Design review of the part built by this model. Coordinates are the model's own, in mm. A direction names the side the tool comes from. Round coordinates to 2 decimals unless told otherwise and drop trailing zeros. Order: outer loops, then holes, each group sorted by start corner. A loop starts at its lowest first (then second) coordinate and runs counter-clockwise, first axis right, second up. Notation, with made-up numbers: M -9.75,29.5 L 33.25,29.5 A16 cw 33.25,46.5 Z; hole C 57,-23 d9. An arc over 180 degrees is marked long. Use a Markdown table: item, result. Add a question column.
(1) For pin 1 (1.3 mm diameter, centred on x = 19, z = 15, fed in from -Y); pin 2 (5 mm diameter, centred on y = -55, z = 13.5, fed in from -X); pin 3 (7 mm diameter, centred on y = -20, z = 6, fed in from -X), all flat-tipped, find the tip position at first contact; note any pin that passes through.
(2) Take a section at D-D (z = 1.5). Write out the cut boundary in (x, y).
(3) Take a section at A-A (z = 11.5). Write out the cut boundary in (x, y), then the cut area to 3 significant figures.
(4) To check wall thickness, follow probe 1 along X at (y, z) = (-6, 17.5); probe 2 along Y at (x, z) = (8, 9.25); probe 3 along Y at (x, z) = (19, 12.75). State the ranges of each line that lie inside material, in increasing order. Write a range as from..to.
(5) Take a section at B-B (x = -12). Write out the cut boundary in (y, z).
(6) Machinability: for faces 1 (the face through (-8.47, -48.65, 4.29)), 2 (the face through (10.631, -13, 11)), 3 (the face through (-33, 11.072, 11)), 4 (the face through (-35.89, 22.67, 11.34)), 5 (the face through (-7, 8, 23)), which of the approach directions +Z, -Z, +X, -X, +Y, -Y give a long, thin tool a straight path to every point of the face, cutting with its end or side? Answer none if there is none.
(7) Take a section at C-C (y = 9.5). Write out the cut boundary in (x, z).
```python
from build123d import *

# Parameters (mm, degrees)
F0_W     = 35
F0_H     = 40
F1_DEPTH = 23
F2_R     = 3
F3_R     = 4
F4_R     = 7
F5_R     = 7.384577
F6_DEPTH = 40


with BuildPart() as f1:
    # F0 (on Top) → F1 (new body)
    with BuildSketch(Plane.XY):
        with Locations((-6.869268, -8.927752)):
            Rectangle(F0_W, F0_H)
        Polygon((19.630732, 31.072248), (-33.369268, 31.072248), (-39.369268, 11.072248), (-24.369268, 11.072248), (10.630732, 11.072248), (25.630732, 11.072248), align=None)
    extrude(amount=F1_DEPTH)

    # F2
    f2_edges = [f1.edges().sort_by_distance(p)[0] for p in [
        (-33.369268, 31.072248, 11.5),
        (19.630732, 31.072248, 11.5),
    ]]
    fillet(f2_edges, radius=F2_R)

    # F3
    f3_edges = [f1.edges().sort_by_distance(p)[0] for p in [
        (-39.369268, 11.072248, 11.5),
        (25.630732, 11.072248, 11.5),
    ]]
    fillet(f3_edges, radius=F3_R)

    # F4
    f4_edges = [f1.edges().sort_by_distance(p)[0] for p in [
        (-24.369268, 11.072248, 11.5),
        (10.630732, 11.072248, 11.5),
    ]]
    fillet(f4_edges, radius=F4_R)

    # F5 (on face) → F6 (join)
    with BuildSketch(Plane.XZ.offset(28.927752)):
        with Locations((-6.869268, 11.5)):
            Circle(F5_R)
    extrude(amount=F6_DEPTH)


solid = f1.part
```
Verdict:
| question | item | result |
|---|---|---|
| 1 | pin 1 | stops at y = 11.07 |
| 1 | pin 2 | stops at x = -14.25 |
| 1 | pin 3 | stops at x = -24.37 |
| 2 | outline | M -37.82,16.22 A4 ccw -33.99,11.07 L -31.37,11.07 A7 cw -24.37,4.07 L -24.37,-28.93 L 10.63,-28.93 L 10.63,4.07 A7 cw 17.63,11.07 L 20.25,11.07 A4 ccw 24.09,16.22 L 20.27,28.93 A3 ccw 17.4,31.07 L -31.14,31.07 A3 ccw -34.01,28.93 Z |
| 3 | outline | M -37.82,16.22 A4 ccw -33.99,11.07 L -31.37,11.07 A7 cw -24.37,4.07 L -24.37,-28.93 L -14.25,-28.93 L -14.25,-68.93 L 0.52,-68.93 L 0.52,-28.93 L 10.63,-28.93 L 10.63,4.07 A7 cw 17.63,11.07 L 20.25,11.07 A4 ccw 24.09,16.22 L 20.27,28.93 A3 ccw 17.4,31.07 L -31.14,31.07 A3 ccw -34.01,28.93 Z |
| 3 | area | 3,180 mm^2 |
| 4 | probe 1 | x = -24.37..10.63 |
| 4 | probe 2 | y = -28.93..31.07 |
| 4 | probe 3 | y = 11.07..30.61 |
| 5 | outline | M -68.93,6.19 L -28.93,6.19 L -28.93,0 L 31.07,0 L 31.07,23 L -28.93,23 L -28.93,16.81 L -68.93,16.81 Z |
| 6 | face 1 | -Y |
| 6 | face 2 | +Z, -Z, +X, -Y |
| 6 | face 3 | +Z, -Z, -X, -Y |
| 6 | face 4 | +Z, -Z, -X, +Y |
| 6 | face 5 | +Z, +X, -X, +Y, -Y |
| 7 | outline | M -26.95,0 L 13.21,0 L 13.21,23 L -26.95,23 Z |
